Here's the drawing with two shaded views (mm, measured from the low corner). I have some questions. Coordinates: 2 decimals unless noted, no trailing zeros. Order: outer loops, then holes, each group sorted by start corner. A loop starts at its lowest first (then second) coordinate and runs counter-clockwise, first axis right, second up. Notation, with made-up numbers: (-3.5, 50) -> (39.5, 50) arc R26 ccw to (39.5, 72) -> close; hole circle Ø9 at (77.5, 63.25). An arc over 180 degrees is marked (long way). One line per item, written item: value. Start each with the question number.
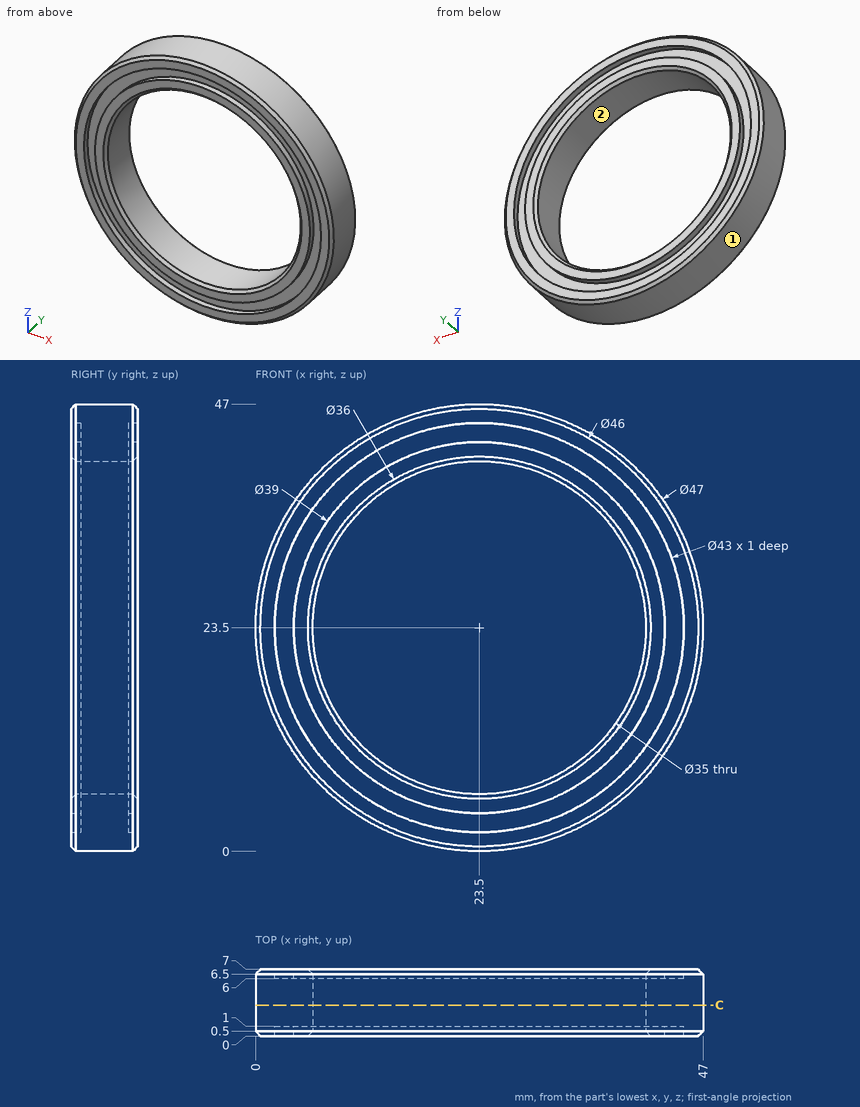
Q1. I need wall thicknesses on line 1 (X direction, y = 0.5, z = 23.5); line 2 (X direction, y = 2.95, z = 23.5); line 3 (X direction, y = 0.3, z = 23.5). Which ranges of each line are inside material? Lowest first, please.
Q2. Imagine slicing it at C-C (y = 3.25). Write out the boundary of the cut face in (x, z), plus the area to 3 significant figures.
Q3. If we mould it in two halves opening along X, with no side actions, what happens to the marked faces 1 and 2? For each: +X half, -X half, draft (parallel to the pull), parting line (faces both ways), or undercut.
Q4. For P1, Ø2, axis at x = 32, y = 1, coming from the +Z side; P2, Ø2, axis at y = 4, z = 25.5, coming from the -X side; P3, Ø1.5, axis at y = 3, z = 12, coming from the +X side, each with a flat end and sliding along its axis, tell me the tip position at first contact or that it passes through.
Completed:
1. line 1: x = 0 to 2, 4 to 6, 41 to 43, 45 to 47
1. line 2: x = 0 to 6, 41 to 47
1. line 3: x = 0.2 to 2, 4 to 5.8, 41.2 to 43, 45 to 46.8
2. outline: circle Ø47 at (23.5, 23.5); hole circle Ø35 at (23.5, 23.5)
2. area: 773 mm2
3. face 1: parting line
3. face 2: undercut
4. P1: stops at z = 45.77
4. P2: stops at x = 0.02
4. P3: stops at x = 44.4
